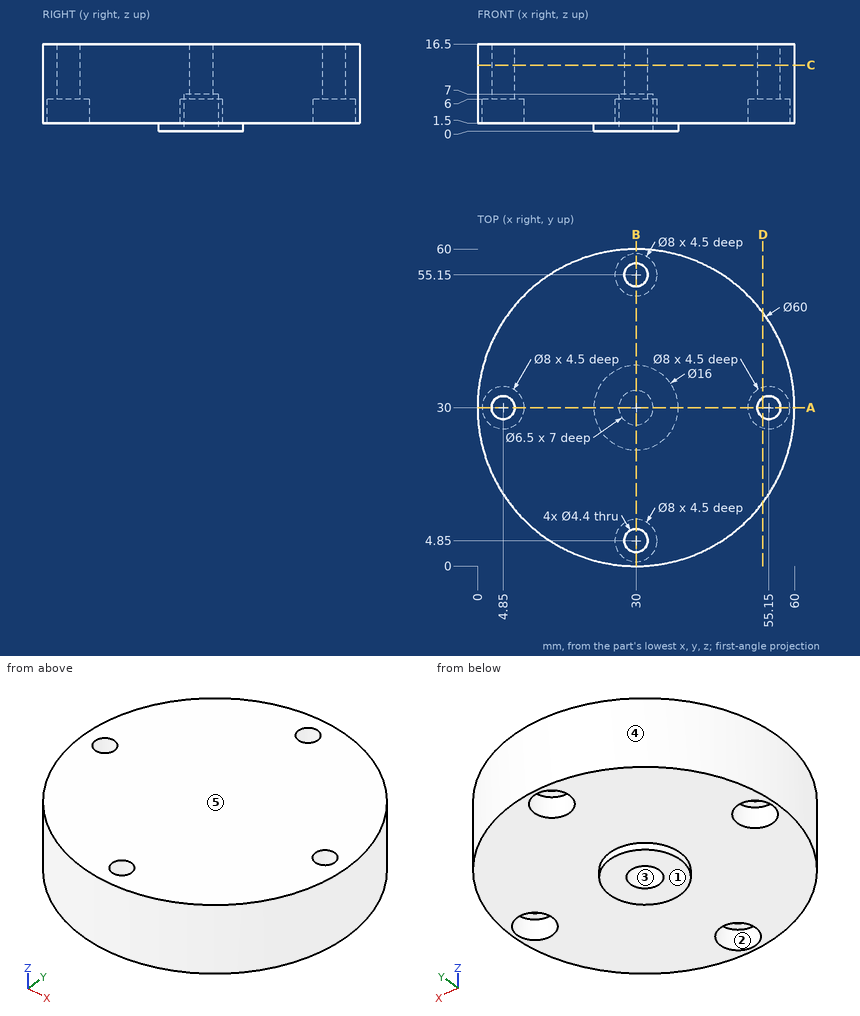
Source: three-view drawing plus pictorial views. Frame: mm from the lowest corner of the part. A direction names the side the tool comes from. Coordinates: 2 decimals unless noted, no trailing zeros. Loops run counter-clockwise (first coordinate to the right, second up) from the corner with the lowest first, then second, coordinate; pieces in that order, holes last. Notation, with made-up numbers: (53.25, -1.5) -> (97.25, -1.5) arc R21 cw to (97.25, 3.5) -> close; hole circle Ø5 at (22.5, 61). An arc over 180 degrees is marked (long way). Write each question's results on one line, items separated by ' | '. Start each with the question number.
Q1. Pin query (flat end, axial travel): pin 1 (2 mm diameter, centred on y = 46, z = 7.5, fed in from +X); pin 2 (8 mm diameter, centred on y = 9, z = 5.5, fed in from -X); pin 3 (4 mm diameter, centred on x = 30, y = 30, fed in from -Z). Return the tip coordinate at first contact, or that it passes through.
Q2. Pull-direction query (Y, two-part tool) for the marked faces 3, 4 and 5; classes: released by +Y, released by -Y, zero draft, split by the parting line, or undercut.
Q3. Section C-C, the plane z = 12.5. Return the cut outline in (x, y).
Q4. Section A-A, the plane y = 30. Return the cut outline in (x, z), plus the area to 3 significant figures.
Q5. Reachability of the marked faces 1 and 2 from +Z, -Z, +X, -X, +Y, -Y: full face, straight path, thin tool, end or side. Return the list, or none.
Q6. Ray query, line 1 (Y direction, x = 30, z = 2.9); line 2 (Y direction, x = 30, z = 14); line 3 (Y direction, x = 28, z = 2). Return the intervals inside material, ascending. Write a range as from..to.
Q7. Section D-D, the plane x = 54. Return the cut outline in (y, z), plus the area to 3 significant figures.
Found:
1) pin 1: x = 55.98 | pin 2: x = 5.28 | pin 3: z = 7
2) face 3: undercut | face 4: split by the parting line | face 5: zero draft
3) outline: circle Ø60 at (30, 30); hole circle Ø4.4 at (4.85, 30); hole circle Ø4.4 at (30, 4.85); hole circle Ø4.4 at (30, 55.15); hole circle Ø4.4 at (55.15, 30)
4) outline: (0, 1.5) -> (0.85, 1.5) -> (0.85, 6) -> (2.65, 6) -> (2.65, 16.5) -> (0, 16.5) -> close; (7.05, 6) -> (8.85, 6) -> (8.85, 1.5) -> (22, 1.5) -> (22, 0) -> (26.75, 0) -> (26.75, 7) -> (33.25, 7) -> (33.25, 0) -> (38, 0) -> (38, 1.5) -> (51.15, 1.5) -> (51.15, 6) -> (52.95, 6) -> (52.95, 16.5) -> (7.05, 16.5) -> close; (57.35, 6) -> (59.15, 6) -> (59.15, 1.5) -> (60, 1.5) -> (60, 16.5) -> (57.35, 16.5) -> close | area: 714 mm2
5) face 1: -Z, +X, -X, +Y, -Y | face 2: -Z
6) line 1: 0..0.85, 8.85..26.75, 33.25..51.15, 59.15..60 | line 2: 0..2.65, 7.05..52.95, 57.35..60 | line 3: 0.07..1.39, 8.31..27.44, 32.56..51.69, 58.61..59.93
7) outline: (12, 1.5) -> (26.17, 1.5) -> (26.17, 6) -> (28.12, 6) -> (28.12, 16.5) -> (12, 16.5) -> close; (31.88, 6) -> (33.83, 6) -> (33.83, 1.5) -> (48, 1.5) -> (48, 16.5) -> (31.88, 16.5) -> close | area: 466 mm2
